Here's how the part is built. I have some questions about the finished solid (model axes, mm). Round coordinates to 2 decimals unless told otherwise and drop trailing zeros. Loops run counter-clockwise (first coordinate to the right, second up) from the corner with the lowest first, then second, coordinate; pieces in that order, holes last. Notation, with made-up numbers: M 72,45 L 127,45 A28 cw 127,84 Z; hole C -4.5,33 d7. An arc over 180 degrees is marked long. Use a Markdown table: item, result.
from build123d import *

# Parameters (mm, degrees)
SKETCH009_W             = 84
SKETCH009_H             = 70
PAD002_DEPTH            = 2
SKETCH010_W             = 2
SKETCH010_H             = 7
PAD003_DEPTH            = 2
SKETCH012_W             = 8
SKETCH012_H             = 6.8
PAD004_DEPTH            = 4
SKETCH013_W             = 7
SKETCH013_H             = 6
PAD005_DEPTH            = 4
SKETCH011_W             = 8
SKETCH011_H             = 6.8
PAD006_DEPTH            = 4
SKETCH014_R             = 1.15
POCKET002_DEPTH         = 81.001
SKETCH016_R             = 1.15
POCKET003_DEPTH         = 8.501
SKETCH018_W             = 11.5
SKETCH018_H             = 11.5
POCKET004_DEPTH         = 5
POCKET005_DEPTH         = 5
POCKET006_DEPTH         = 5
SKETCH022_W             = 9
SKETCH022_H             = 10
POCKET007_DEPTH         = 0.4
FILLET_R                = 3
BODY002_PITCH_ANGLE     = -90
BODY002_PLACEMENT_ANGLE = 90
PAD001_DEPTH            = 35
SKETCH007_W             = 11.5
SKETCH007_H             = 11.5
POCKET001_DEPTH         = 13
FILLET001_R             = 3
SKETCH025_W             = 6.5
SKETCH025_H             = 9
SKETCH025_W_2           = 9
SKETCH025_H_2           = 6.5
POCKET008_DEPTH         = 8


with BuildPart() as back:
    # Sketch009 → Pad002 (new body)
    with BuildSketch(Plane.XY):
        Rectangle(SKETCH009_W, SKETCH009_H)
    extrude(amount=PAD002_DEPTH)

    # Sketch010 (on Face6 of Pad002) → Pad003 (join)
    with BuildSketch(Plane.XY.offset(2)):
        with Locations((-38, -1)):
            Rectangle(SKETCH010_W, SKETCH010_H)
        Polygon((-21, 32), (39, 32), (39, -4), (37, -4), (37, 30), (-21, 30), align=None)
    extrude(amount=PAD003_DEPTH)

    # Sketch012 (on Face15 of Pad003) → Pad004 (join)
    with BuildSketch(Plane.YZ.offset(39)):
        with Locations((0, 5.4)):
            Rectangle(SKETCH012_W, SKETCH012_H)
    extrude(amount=-PAD004_DEPTH)

    # Sketch013 (on Face9 of Pad004) → Pad005 (join)
    with BuildSketch(Plane(origin=(-39, 0, 0), x_dir=(0, -1, 0), z_dir=(-1, 0, 0))):
        with Locations((1, 5)):
            Rectangle(SKETCH013_W, SKETCH013_H)
    extrude(amount=-PAD005_DEPTH)

    # Sketch011 (on Face16 of Pad003) → Pad006 (join)
    with BuildSketch(Plane(origin=(0, 32, 0), x_dir=(-1, 0, 0), z_dir=(0, 1, 0))):
        with Locations((-29, 5.4)):
            Rectangle(SKETCH011_W, SKETCH011_H)
        with Locations((14, 5.4)):
            Rectangle(SKETCH011_W, SKETCH011_H)
    extrude(amount=-PAD006_DEPTH)

    # Sketch014 (on Face44 of Pad006) → Pocket002 (cut, through all)
    with BuildSketch(Plane.YZ.offset(39)):
        with Locations((0, 5)):
            Circle(SKETCH014_R)
    extrude(amount=-POCKET002_DEPTH, mode=Mode.SUBTRACT)

    # Sketch016 → Pocket003 (cut, through all)
    with BuildSketch(Plane.XZ.offset(-26.5)):
        with Locations((-13, 5)):
            Circle(SKETCH016_R)
        with Locations((30, 5)):
            Circle(SKETCH016_R)
    extrude(amount=-POCKET003_DEPTH, mode=Mode.SUBTRACT)

    # Sketch018 (on Face5 of Pocket003) → Pocket004 (cut)
    with BuildSketch(Plane.XY.offset(2)):
        with Locations((0, 17.75)):
            Rectangle(SKETCH018_W, SKETCH018_H)
    extrude(amount=-POCKET004_DEPTH, mode=Mode.SUBTRACT)

    # Sketch019 (on Face31 of Pocket004) → Pocket005 (cut)
    with BuildSketch(Plane.XZ.offset(-28)):
        Polygon((29.125944, 9.042901), (33.258869, 4.499726), (33.258869, 9.042901), align=None)
    extrude(amount=-POCKET005_DEPTH, mode=Mode.SUBTRACT)

    # Sketch020 (on Face36 of Pocket005) → Pocket006 (cut)
    with BuildSketch(Plane(origin=(35, 0, 0), x_dir=(0, -1, 0), z_dir=(-1, 0, 0))):
        Polygon((2.77547, 8.938441), (6.386171, 3.079567), (6.386171, 8.938441), align=None)
    extrude(amount=-POCKET006_DEPTH, mode=Mode.SUBTRACT)

    # Sketch022 (on Face5 of Pocket005) → Pocket007 (cut)
    with BuildSketch(Plane.XY.offset(2)):
        with Locations((-30.3, 30)):
            Rectangle(SKETCH022_W, SKETCH022_H)
    extrude(amount=-POCKET007_DEPTH, mode=Mode.SUBTRACT)

    # Fillet
    fillet_edges = [back.edges().sort_by_distance(p)[0] for p in [
        (42, 35, 1),
        (-42, 35, 1),
    ]]
    fillet(fillet_edges, radius=FILLET_R)


with BuildPart() as back_1:
    # Body002 pitch: moved
    add(back.part.rotate(Axis((0, 0, 0), (0, 1, 0)), BODY002_PITCH_ANGLE))


with BuildPart() as back_2:
    # Body002 placement: moved
    add(back_1.part.rotate(Axis((0, 0, 0), (0, 0, 1)), BODY002_PLACEMENT_ANGLE))


with BuildPart() as curve:
    # Sketch006 → Pad001 (new body, symmetric)
    with BuildSketch(Plane(origin=(0, 0, 0), x_dir=(0, 0, -1), z_dir=(1, 0, 0))):
        with BuildLine():
            ThreePointArc((-42, 2.4), (0, 1.334097), (42, 2.4))
            Line((42, -0.1), (42, 2.4))
            Line((-42, -0.1), (42, -0.1))
            Line((-42, 2.4), (-42, -0.1))
        make_face()
    extrude(amount=PAD001_DEPTH, both=True)

    # Sketch007 (on Face3 of Pad001) → Pocket001 (cut)
    with BuildSketch(Plane.XZ.offset(0.1)):
        with Locations((-17.75, 0)):
            Rectangle(SKETCH007_W, SKETCH007_H)
    extrude(amount=-POCKET001_DEPTH, mode=Mode.SUBTRACT)

    # Fillet001
    fillet001_edges = [curve.edges().sort_by_distance(p)[0] for p in [
        (-35, 1.15, -42),
        (-35, 1.15, 42),
    ]]
    fillet(fillet001_edges, radius=FILLET001_R)

    # Boolean: union Back
    add(back_2.part)

    # Sketch025 (on Face32 of Boolean) → Pocket008 (cut, symmetric)
    with BuildSketch(Plane.XZ.offset(2)):
        with Locations((-28.75, 0)):
            Rectangle(SKETCH025_W, SKETCH025_H)
        with Locations((-15.55, 13.625)):
            Rectangle(SKETCH025_W_2, SKETCH025_H_2)
        with Locations((-2.05, 0)):
            Rectangle(SKETCH025_W, SKETCH025_H)
        with Locations((-15.55, -13.625)):
            Rectangle(SKETCH025_W_2, SKETCH025_H_2)
    extrude(amount=POCKET008_DEPTH, both=True, mode=Mode.SUBTRACT)


solid = curve.part
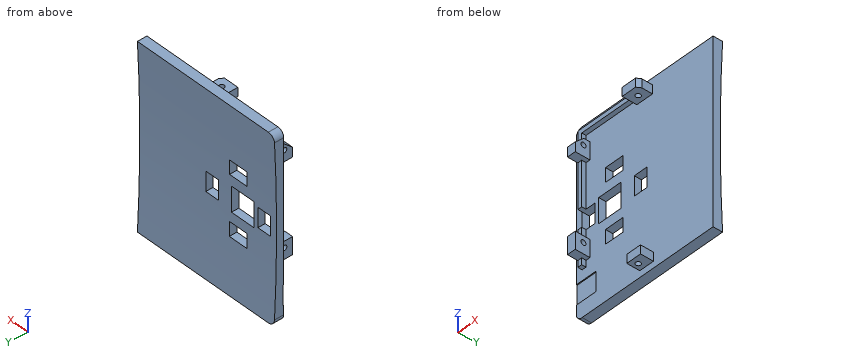
1. Imagine slicing it at D-D, the plane x = 0. Write out the boundary of the cut face in (y, z).
Answer sheet:
| item | result |
|---|---|
| outline | M -8.8,35 L -6.15,35 L -6.15,39 L -8.8,39 Z; M -8,-39 L -6.15,-39 L -6.15,-35 L -8,-35 Z; M -3.85,-39 L -2,-39 L -2,-42 L 2.4,-42 A828 cw 1.35,-4.5 L -2,-4.5 L -2,-35 L -3.85,-35 Z; M -3.85,35 L -2,35 L -2,4.5 L 1.35,4.5 A828 cw 2.4,42 L -2,42 L -2,39 L -3.85,39 Z |
2. For pin 1 Ø6.5 at (x, y) = (-0.5, -4) entering from -Z; pin 2 Ø2 at (y, z) = (-4.5, 37) entering from -X; pin 3 Ø2 at (x, y) = (-30, -4) entering from -Z; pin 4 Ø1.2 at (y, z) = (-3.5, 38) entering from +X, each with a flat end and sliding along its axis, tell me the tip position at first contact or that it passes through.
Answer sheet:
| item | result |
|---|---|
| pin 1 | z = -42 |
| pin 2 | x = -32 |
| pin 3 | z = -21 |
| pin 4 | x = 4 |
3. I need wall thicknesses on probe 1 along Z at (x, y) = (-28, 0); probe 2 along X at (y, z) = (-4.75, -10.5); probe 3 along X at (y, z) = (-5, -38.2). Which ranges of each line are inside material? Lowest first, please. Write a range as from..to.
Answer sheet:
| item | result |
|---|---|
| probe 1 | -42..-4.5, 4.5..42 |
| probe 2 | -32..-28 |
| probe 3 | -2.5..-1.15, 1.15..4.5 |
4. Imagine slicing it at C-C, the plane z = -13. Write out the boundary of the cut face in (x, y).
Answer sheet:
| item | result |
|---|---|
| outline | M -35,-2 L -32,-2 L -32,-3.85 L -28,-3.85 L -28,-2 L -20.05,-2 L -20.05,1.44 L -35,1.44 Z; M -32,-8.8 L -28,-8.8 L -28,-6.15 L -32,-6.15 Z; M -11.05,-2 L 35,-2 L 35,1.44 L -11.05,1.44 Z |
5. Imagine slicing it at B-B, the plane y = -0.5. Write out the boundary of the cut face in (x, z) (3 decimals), then the cut area to 3 significant figures.
Answer sheet:
| item | result |
|---|---|
| outline | M -35,-39 A3 ccw -32,-42 L 35,-42 L 35,42 L -32,42 A3 ccw -35,39 Z; hole M -32,-4.5 L -25.5,-4.5 L -25.5,4.5 L -32,4.5 Z; hole M -23.5,-5.75 L -12,-5.75 L -12,5.75 L -23.5,5.75 Z; hole M -20.05,-16.875 L -11.05,-16.875 L -11.05,-10.375 L -20.05,-10.375 Z; hole M -20.05,10.375 L -11.05,10.375 L -11.05,16.875 L -20.05,16.875 Z; hole M -5.3,-4.5 L 1.2,-4.5 L 1.2,4.5 L -5.3,4.5 Z |
| area | 5,510 mm2 |
6. Imagine slicing it at A-A, the plane x = -18. Write out the boundary of the cut face in (y, z) (3 decimals), then the cut area to 3 significant figures.
Answer sheet:
| item | result |
|---|---|
| outline | M -4,37 L -2,37 L -2,16.875 L 1.506,16.875 A828 cw 2.4,42 L -2,42 L -2,39 L -4,39 Z; M -2,-42 L 2.4,-42 A828 cw 1.506,-16.875 L -2,-16.875 Z; M -2,-10.375 L 1.399,-10.375 A828 cw 1.354,-5.75 L -2,-5.75 Z; M -2,5.75 L 1.354,5.75 A828 cw 1.399,10.375 L -2,10.375 Z |
| area | 231 mm2 |
